```python
from build123d import *

# Parameters (mm, degrees)
SKETCH_1_R            = 4.5
EXTRUDE_1_DEPTH       = 34
SKETCH_2_R            = 4
EXTRUDE_2_DEPTH       = 3
SKETCH_3_R            = 4
EXTRUDE_3_DEPTH       = 23
SKETCH_7_W            = 1.79623407
SKETCH_7_H            = 9.81557087
SKETCH_7_W_2          = 2.958566665
SKETCH_7_H_2          = 10.839995421
CUT_EXTRUDE_14_DEPTH  = 4
HOLE_WIZARD_M53_D     = 5.2
HOLE_WIZARD_M53_DEPTH = 13
HOLE_WIZARD_M53_TIP   = 1.562237609
SKETCH_16_R           = 10.346676453
SKETCH_16_W           = 7
SKETCH_16_H           = 7
CUT_EXTRUDE_15_DEPTH  = 10


# Read off the part's stored shape, not the designer's step: the extrude step
with BuildPart() as part:
    # Sketch 1 → Extrude 1 (new body)
    with BuildSketch(Plane.XY):
        Circle(SKETCH_1_R)
    extrude(amount=EXTRUDE_1_DEPTH)

    # Sketch 2 → Extrude 2 (add)
    with BuildSketch(Plane.XY.offset(34)):
        Circle(SKETCH_2_R)
    extrude(amount=EXTRUDE_2_DEPTH)

    # Sketch 3 → Extrude 3 (add)
    # profile 1 of 2: a face of its own
    with BuildSketch(Plane.XY.offset(37)):
        with BuildLine():
            ThreePointArc((6, 3.605551275), (3.446820352, 6.092571663), (0, 7))
            ThreePointArc((0, 7), (-3.446820352, 6.092571663), (-6, 3.605551275))
            Line((-6, 3.605551275), (-6, -3.605551275))
            ThreePointArc((-6, -3.605551275), (-3.446820352, -6.092571663), (0, -7))
            ThreePointArc((0, -7), (3.446820352, -6.092571663), (6, -3.605551275))
            Line((6, -3.605551275), (6, 3.605551275))
        make_face()
        Circle(SKETCH_3_R, mode=Mode.SUBTRACT)
    # profile 2 of 2: a face of its own
    with BuildSketch(Plane.XY.offset(37)):
        Circle(SKETCH_3_R)
    extrude(amount=EXTRUDE_3_DEPTH)

    # Extrude 4 outline → Extrude 4 (revolve)
    with BuildSketch(Plane(origin=(0.00751481, -0.003794932, 0), x_dir=(1, 0, 0), z_dir=(0, -1, 0))):
        Polygon((2, 70), (0, 70), (0, 60), (7.095254495, 60), align=None)
    revolve(axis=Axis((0.00751481, -0.003794932, 0), (0, 0, 1)))

    # Sketch 7 → Cut-Extrude 14 (cut)
    with BuildSketch(Plane(origin=(0, 0, 60), x_dir=(-1, 0, 0), z_dir=(0, 0, -1))):
        with Locations((-6.898117035, 0.517903439)):
            Rectangle(SKETCH_7_W, SKETCH_7_H)
        with Locations((7.479283333, -1.183503448)):
            Rectangle(SKETCH_7_W_2, SKETCH_7_H_2)
    extrude(amount=-CUT_EXTRUDE_14_DEPTH, mode=Mode.SUBTRACT)

    # Hole Wizard M53
    with Locations(Plane(origin=(0, 0, 0), x_dir=(-1, 0, 0), z_dir=(0, 0, -1))):
        with Locations((0, 0)):
            Hole(HOLE_WIZARD_M53_D / 2, depth=HOLE_WIZARD_M53_DEPTH)
            with Locations((0, 0, -(HOLE_WIZARD_M53_DEPTH + HOLE_WIZARD_M53_TIP / 2))):  # 118° drill point
                Cone(0, HOLE_WIZARD_M53_D / 2, HOLE_WIZARD_M53_TIP, mode=Mode.SUBTRACT)

    # Sketch 16 → Cut-Extrude 15 (cut)
    with BuildSketch(Plane(origin=(0, 0, 0), x_dir=(-1, 0, 0), z_dir=(0, 0, -1))):
        Circle(SKETCH_16_R)
        Rectangle(SKETCH_16_W, SKETCH_16_H, mode=Mode.SUBTRACT)
    extrude(amount=-CUT_EXTRUDE_15_DEPTH, mode=Mode.SUBTRACT)


solid = part.part
```
Geometry: final body of the model. Coordinates: model frame, mm. A direction names the side the tool comes from. Coordinates: 2 decimals unless noted, no trailing zeros. Order: outer loops, then holes, each group sorted by start corner. A loop starts at its lowest first (then second) coordinate and runs counter-clockwise, first axis right, second up. Notation, with made-up numbers: (-6.5, 33) - (20.5, 33) arc R27 cw to (20.5, 50) - close; hole circle Ø3 at (74, -12). An arc over 180 degrees is marked (long way). Return JSON: item names as keys, results as strings. Group by question number.
1. Material intervals for line 1 along Y through (x, z) = (0, 5); line 2 along X through (y, z) = (-3.5, 63.5), sorted ascending. Write a range as [from, to].
2. Cut plane A-A (z = 55.5). Output: boundary loops of the cut face in (x, y), plus the area to 3 significant figures.
3. Cut plane B-B (z = 32). Output: boundary loops of the cut face in (x, y), plus the area to 3 significant figures.
4. Set-up query: faces 5 (the face through (0, -3.5, 5)), 6 (the face through (-3, -3, 34)), 7 (the face through (0, 3.5, 5)), 8 (the face through (-3.5, 0, 5)), 9 (the face through (-3.32, 3.04, 20.54)). Return all of +Z, -Z, +X, -X, +Y, -Y with unobstructed straight access to the full face (end or side cutting, diameter ignored); none if empty.
5. Pin query (flat end, axial travel): pin 1 (3 mm diameter, centred on y = 0.5, z = 3.5, fed in from +X); pin 2 (0.5 mm diameter, centred on x = -0.5, y = -4, fed in from -Z); pin 3 (1.7 mm diameter, centred on x = -2.5, y = -5, fed in from -Z). Return the tip coordinate at first contact, or that it passes through.
6. Pull-direction query (X, two-part tool) for faces 1 (the face through (0.33, 0.31, 14.29)), 2 (the face through (6, 0, 49)), 3 (the face through (-0.338, 2.578, 6.591)), 4 (the face through (-0.867, -3.905, 35.479)); classes: pulls with the +X half, pulls with the -X half, needs draft (parallel to the pull), parting line crosses it, or undercut.
Resolved:
{
 "1": {"line 1": "y = [-3.5, -2.6], [2.6, 3.5]", "line 2": "x = [-3.99, 4.01]"},
 "2": {"outline": "(-6, -3.61) arc R7 ccw to (6, -3.61) - (6, 3.61) arc R7 ccw to (-6, 3.61) - close", "area": "144 mm²"},
 "3": {"outline": "circle Ø9 at (0, 0)", "area": "63.6 mm²"},
 "4": {"face 5": "-Z, +X, -X, -Y", "face 6": "none", "face 7": "-Z, +X, -X, +Y", "face 8": "-Z, -X, +Y, -Y", "face 9": "-Z"},
 "5": {"pin 1": "stops at x = 3.5", "pin 2": "stops at z = 10", "pin 3": "stops at z = 37"},
 "6": {"face 1": "undercut", "face 2": "pulls with the +X half", "face 3": "undercut", "face 4": "parting line crosses it"}
}
